from build123d import *

# Parameters (mm, degrees)
EXTRUDE_1_DEPTH     = 20
FILLET_1_R          = 5
SKETCH_2_R          = 1
CUT_EXTRUDE_1_DEPTH = 10
SKETCH_3_R          = 10
CUT_EXTRUDE_2_DEPTH = 40


with BuildPart() as part:
    # 草图1 → 凸台-拉伸1 (new body)
    with BuildSketch(Plane.XY):
        with BuildLine():
            Line((0, 29), (0, 25))
            Line((0, 25), (-4.6, 25))
            ThreePointArc((-4.6, 25), (-9.6, 20), (-4.6, 15))
            Line((-4.6, 15), (0, 15))
            Line((0, 15), (0, -15))
            Line((0, -15), (-4.6, -15))
            ThreePointArc((-4.6, -15), (-9.6, -20), (-4.6, -25))
            Line((-4.6, -25), (0, -25))
            Line((0, -25), (0, -29))
            Line((0, -29), (-14, -29))
            Line((-14, -29), (-14, 29))
            Line((-14, 29), (0, 29))
        make_face()
    extrude(amount=EXTRUDE_1_DEPTH)

    # 圆角1
    fillet_1_edges = [part.edges().sort_by_distance(p)[0] for p in [
        (-14, -29, 10),
        (-14, 29, 10),
    ]]
    fillet(fillet_1_edges, radius=FILLET_1_R)

    # 草图2 → 切除-拉伸1 (cut)
    with BuildSketch(Plane(origin=(0, 0, 0), x_dir=(0, 0, -1), z_dir=(1, 0, 0))):
        with Locations((-16, 27.2)):
            Circle(SKETCH_2_R)
        with Locations((-4, 27.2)):
            Circle(SKETCH_2_R)
        with Locations((-10, 11)):
            Circle(SKETCH_2_R)
        with Locations((-10, -11)):
            Circle(SKETCH_2_R)
        with Locations((-15, -27)):
            Circle(SKETCH_2_R)
        with Locations((-5, -27)):
            Circle(SKETCH_2_R)
    extrude(amount=-CUT_EXTRUDE_1_DEPTH, mode=Mode.SUBTRACT)

    # 草图3 → 切除-拉伸2 (cut)
    with BuildSketch(Plane.XY.offset(20)):
        with Locations((-14, 0)):
            Circle(SKETCH_3_R)
    extrude(amount=-CUT_EXTRUDE_2_DEPTH, mode=Mode.SUBTRACT)


solid = part.part
Input: part model. Units: mm. Frame: model coordinates. A direction names the side the tool comes from. Coordinates: 2 decimals unless noted, no trailing zeros. Write each loop counter-clockwise with the first axis right and the second up, starting at its lowest first coordinate (ties: lowest second). Pieces come first, ordered by that corner, then holes. Notation, with made-up numbers: M 48,47.5 L 66,47.5 A21 ccw 66,57.5 Z; hole C 80,56 d6. An arc over 180 degrees is marked long. Answer as a JSON object with one key per item and string values. Group by question number.
(1) Section D-D on y = -27. Output: boundary loops of the cut face in (x, z).
(2) Contact query for flat-ended pins moving along their axis: P1, Ø1.5, axis at y = 6.5, z = 9, coming from the -X side; P2, Ø6, axis at x = -4.5, y = 20, coming from the +Z side; P3, Ø0.6, axis at y = -27, z = 4.5, coming from the +X side; P4, Ø1.8, axis at y = -27, z = 5, coming from the -X side. Output: stop coordinate, or through.
(3) Set-up query: faces 1 (the face through (-4.93, -26.324, 5.737)), 2 (the face through (-2, -25, 10)), 3 (the face through (-14, -17, 10)). Return all of +Z, -Z, +X, -X, +Y, -Y with unobstructed straight access to the full face (end or side cutting, diameter ignored); none if empty.
(4) Ray query, line 1 along Y through (x, z) = (-2, 6.5); line 2 along Y through (x, z) = (-4.75, 13); line 3 along Y through (x, z) = (-5.5, 5.25). Return the intervals inside material, ascending. Write a range as [from, to].
(5) Section B-B on z = 12.75. Output: boundary loops of the cut face in (x, y), plus the area to 3 significant figures.
(6) Section C-C on y = -11. Output: boundary loops of the cut face in (x, z).
(7) Section A-A on x = -2. Give the number of separate pieces and of enclosed holes in the cut face, plus the area to 3 significant figures.
Result set:
{
 "1": {"outline": "M -13,0 L 0,0 L 0,4 L -10,4 L -10,6 L 0,6 L 0,14 L -10,14 L -10,16 L 0,16 L 0,20 L -13,20 Z"},
 "2": {"P1": "stops at x = -7.11", "P2": "passes through", "P3": "stops at x = -10", "P4": "stops at x = -13.54"},
 "3": {"face 1": "+X", "face 2": "+Z, -Z, +X", "face 3": "+Z, -Z, -X, +Y, -Y"},
 "4": {"line 1": "y = [-29, -25], [-15, 15], [25, 29]", "line 2": "y = [-29, -25], [-15, -3.8], [3.8, 15], [25, 29]", "line 3": "y = [-29, -27.97], [-26.03, -24.92], [-15.08, -5.27], [5.27, 15.08], [24.92, 29]"},
 "5": {"outline": "M -14,-24 A5 ccw -9,-29 L 0,-29 L 0,-25 L -4.6,-25 A5 cw -4.6,-15 L 0,-15 L 0,15 L -4.6,15 A5 cw -4.6,25 L 0,25 L 0,29 L -9,29 A5 ccw -14,24 L -14,10 A10 cw -14,-10 Z", "area": "474 mm2"},
 "6": {"outline": "M -14,0 L 0,0 L 0,9 L -10,9 L -10,11 L 0,11 L 0,20 L -14,20 Z"},
 "7": {"separate pieces": "3", "enclosed holes": "6", "area": "741 mm2"}
}
